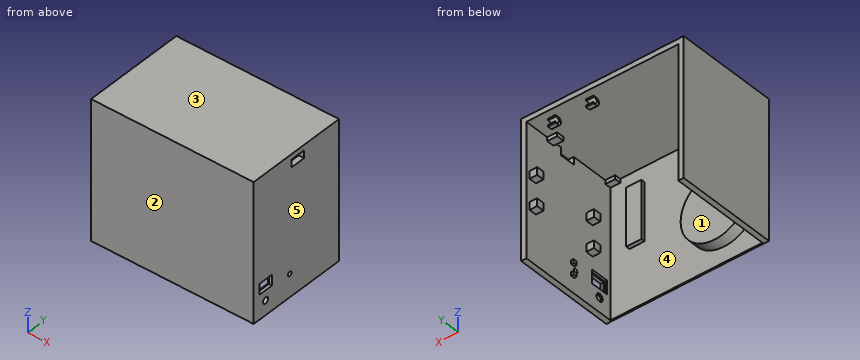
Autodesk Inventor part; units mm, degrees
ref_plane "YZ Plane" through (0, 0, 0) normal (1, 0, 0) x (0, 1, 0)
ref_plane "XY Plane" through (0, 0, 0) normal (0, 0, 1) x (1, 0, 0)
sketch "Boceto1" plane through (0, 0, 0) normal (1, 0, 0) x (0, 1, 0)
  line L0 (135, 82) -> (0, 82)
  line L1 (0, 82) -> (0, -100)
  line L2 (0, -100) -> (135, -100)
  line L3 (135, -100) -> (135, 82)
  line L4 (135, 82) -> (0, -100) construction
  line L5 (0, 82) -> (135, -100) construction
  point P0 (0, 0)
  point P1 (67.5, -9)
  dimension "d0" = 182
  dimension "d1" = 135
  dimension "d2" = 100
extrude "Extrusión1" add sketch "Boceto1" against normal blind 214
sketch "Boceto2" plane through (-214, 0, 0) normal (-1, 0, 0) x (0, 0, 1)
  line L0 (82, 135) -> (-100, 135)
  line L1 (-93, 2) -> (75, 2)
  line L2 (75, 2) -> (75, 135)
  line L3 (75, 135) -> (-93, 135)
  line L4 (-93, 135) -> (-93, 2)
  line L5 (-93, 2) -> (75, 135) construction
  line L6 (75, 2) -> (-93, 135) construction
  line L7 (-100, 0) -> (82, 0)
  line L8 (82, 0) -> (82, 135)
  line L9 (-100, 135) -> (-100, 0)
  point P0 (0, 0)
  point P1 (-9, 68.5)
  point P2 (-93, 135)
  dimension "d5" = 2
  dimension "d6" = 7
  dimension "d7" = 7
extrude "Extrusión2" cut sketch "Boceto2" against normal blind 207 contours L2 L1 L4 L0
sketch "Boceto3" plane through (0, 0, 82) normal (0, 0, 1) x (1, 0, 0)
  line L0 (-20, 0) -> (0, 0)
  line L1 (0, 0) -> (0, 10)
  line L2 (0, 10) -> (-20, 10)
  line L3 (-20, 10) -> (-20, 0)
  line L4 (-20, 0) -> (0, 10) construction
  line L5 (0, 0) -> (-20, 10) construction
  line L6 (-214, 0) -> (-194, 0)
  line L7 (-194, 0) -> (-194, 10)
  line L8 (-194, 10) -> (-214, 10)
  line L9 (-214, 10) -> (-214, 0)
  line L10 (-214, 0) -> (-194, 10) construction
  line L11 (-194, 0) -> (-214, 10) construction
  line L12 (-20, 92) -> (0, 92)
  line L13 (0, 92) -> (0, 102)
  line L14 (0, 102) -> (-20, 102)
  line L15 (-20, 102) -> (-20, 92)
  line L16 (-20, 92) -> (0, 102) construction
  line L17 (0, 92) -> (-20, 102) construction
  line L18 (-214, 0) -> (-214, 135)
  line L19 (0, 135) -> (0, 0)
  line L20 (0, 0) -> (-214, 0)
  line L21 (-214, 92) -> (-194, 92)
  line L22 (-194, 92) -> (-194, 102)
  line L23 (-194, 102) -> (-214, 102)
  line L24 (-214, 102) -> (-214, 92)
  line L25 (-214, 92) -> (-194, 102) construction
  line L26 (-194, 92) -> (-214, 102) construction
  line L27 (-214, 2) -> (-7, 2)
  point P0 (-10, 5)
  point P1 (-204, 5)
  point P2 (-10, 97)
  point P3 (-204, 97)
  point P4 (-10, 0)
  dimension "d10" = 20
  dimension "d11" = 10
  dimension "d13" = 10
  dimension "d14" = 20
  dimension "d65" = 100
extrude "Extrusión3" add sketch "Boceto3" against normal blind 12 contours L3 L2 L1 L0 | L18 L23 L22 L21 | L12 L15 L14 L13 | L6 L9 L27 L7 | L27 L9 L8 L7
sketch "Sketch4" plane through (0, 0, 0) normal (1, 0, 0) x (0, 0, -1)
  line L0 (-82, 0) -> (-82, 135)
  line L1 (-100, 90) -> (-100, 60)
  line L2 (-82, 0) -> (100, 0)
  line L3 (-75, 60) -> (-65, 60)
  line L4 (-65, 60) -> (-65, 80)
  line L5 (-65, 80) -> (-75, 80)
  line L6 (-75, 80) -> (-75, 60)
  line L7 (-75, 60) -> (-65, 80) construction
  line L8 (-65, 60) -> (-75, 80) construction
  point P0 (0, 0)
  point P1 (-70, 70)
  point P2 (-70, 60)
  dimension "d43" = 17
  dimension "d44" = 7
  dimension "d45" = 20
  dimension "d46" = 60
extrude "Extrusion4" cut sketch "Sketch4" against normal up to next
sketch "Sketch5" plane through (-7, 0, 0) normal (-1, 0, 0) x (0, 0, 1)
  line L0 (-35, 130) -> (-25, 130)
  line L1 (-25, 130) -> (-25, 120)
  line L2 (-25, 120) -> (-35, 120)
  line L3 (-35, 120) -> (-35, 130)
  line L4 (5, 130) -> (15, 130)
  line L5 (15, 130) -> (15, 120)
  line L6 (15, 120) -> (5, 120)
  line L7 (5, 120) -> (5, 130)
  line L8 (-35, 40) -> (-25, 40)
  line L9 (-25, 40) -> (-25, 30)
  line L10 (-25, 30) -> (-35, 30)
  line L11 (-35, 30) -> (-35, 40)
  line L12 (15, 40) -> (5, 40)
  line L13 (5, 40) -> (5, 30)
  line L14 (5, 30) -> (15, 30)
  line L15 (15, 30) -> (15, 40)
  line L16 (-93, 135) -> (75, 135)
  line L17 (75, 135) -> (75, 102)
  line L18 (70, 2) -> (-93, 2)
  line L19 (75, 92) -> (75, 10)
  point P0 (0, 0)
  point P1 (-30, 130)
  point P2 (-30, 30)
  point P3 (10, 130)
  point P4 (15, 125)
  dimension "d25" = 10
  dimension "d26" = 10
  dimension "d27" = 10
  dimension "d28" = 10
  dimension "d29" = 100
  dimension "d31" = 5
  dimension "d32" = 60
  dimension "d77" = 50
extrude "Extrusion5" add sketch "Sketch5" along normal blind 10
sketch "Sketch8" plane through (-7, 135, 75) normal (0, 0, -1) x (-1, 0, 0)
  line L0 (20, -20) -> (30, -20)
  line L1 (30, -20) -> (30, -10)
  line L2 (30, -10) -> (20, -10)
  line L3 (20, -10) -> (20, -20)
  line L4 (20, -20) -> (30, -10) construction
  line L5 (30, -20) -> (20, -10) construction
  line L6 (70, -20) -> (80, -20)
  line L7 (80, -20) -> (80, -10)
  line L8 (80, -10) -> (70, -10)
  line L9 (70, -10) -> (70, -20)
  line L10 (70, -20) -> (80, -10) construction
  line L11 (80, -20) -> (70, -10) construction
  line L12 (0, 0) -> (207, 0)
  line L13 (0, 0) -> (0, -33)
  point P0 (-7, -135)
  point P1 (25, -15)
  point P2 (75, -15)
  dimension "d47" = 10
  dimension "d48" = 10
  dimension "d49" = 10
  dimension "d50" = 10
  dimension "d51" = 50
  dimension "d52" = 10
  dimension "d53" = 20
extrude "Extrusion6" add sketch "Sketch8" along normal blind 10
sketch "Sketch9" plane through (-7, 0, 0) normal (-1, 0, 0) x (0, 0, 1)
  line L0 (-68, 9) -> (-54, 9)
  line L1 (-54, 9) -> (-54, 29)
  line L2 (-54, 29) -> (-68, 29)
  line L3 (-68, 29) -> (-68, 9)
  line L4 (-68, 9) -> (-54, 29) construction
  line L5 (-54, 9) -> (-68, 29) construction
  line L6 (70, 2) -> (-93, 2)
  line L7 (-93, 2) -> (-93, 135)
  circle A0 centre (-81, 19) radius 4
  point P0 (0, 0)
  point P1 (-61, 19)
  dimension "d56" = 20
  dimension "d57" = 14
  dimension "d58" = 7
  dimension "d59" = 25
  dimension "d60" = 8
  dimension "d61" = 20
  dimension "d62" = 17
extrude "Extrusion7" cut sketch "Sketch9" against normal up to next
sketch "Sketch10" plane through (-87, 115, 75) normal (-1, 0, 0) x (0, 0, 1)
  line L0 (0, 10) -> (-10, 10)
  arc A0 (-8, 10) -> (-2, 10) centre (-5, 8.1972) ccw
  line L1 (0, 20) -> (0, -13)
  point P0 (-75, -115)
  dimension "d66" = 3.5
  dimension "d67" = 2
  dimension "d68" = 2
extrude "Extrusion8" cut sketch "Sketch10" against normal up to surface (60 mm away)
sketch "Sketch11" plane through (-87, 115, 75) normal (-1, 0, 0) x (0, 0, 1)
  line L0 (-10, 10) -> (-10, 0)
  line L1 (0, 0) -> (0, 10)
  arc A0 (-10, 4.322) -> (0, 4.0877) centre (-4.9301, 7.1893) ccw
  line L2 (-10, 4.322) -> (-10, 0)
  line L3 (0, 0) -> (-10, 0)
  line L4 (0, 0) -> (0, 4.0877)
  line L5 (-10, 4.322) -> (-10, 0)
  line L6 (0, 0) -> (0, 4.0877)
  line L7 (-10, 4.322) -> (-10, 0)
  line L8 (0, 0) -> (0, 4.0877)
  line L9 (-10, 4.322) -> (-10, 0)
  line L10 (0, 0) -> (0, 4.0877)
  point P0 (-75, -115)
  point P1 (-5, 0)
  point P2 (-5.0665, 1.3663)
  dimension "d71" = 5.8246
  dimension "d73" = 4.322
  dimension "d74" = 1.3663
extrude "Extrusion9" cut sketch "Sketch11" against normal up to surface (60 mm away)
sketch "Sketch12" plane through (-214, 2, -93) normal (0, 1, 0) x (1, 0, 0)
  line L0 (162, -72) -> (182, -72)
  line L1 (182, -72) -> (182, -148)
  line L2 (182, -148) -> (162, -148)
  line L3 (162, -148) -> (162, -72)
  line L4 (162, -72) -> (182, -148) construction
  line L5 (182, -72) -> (162, -148) construction
  line L6 (207, 0) -> (207, -168)
  line L7 (207, -168) -> (0, -168)
  point P0 (214, -93)
  point P1 (172, -110)
  dimension "d78" = 76
  dimension "d79" = 20
  dimension "d80" = 25
  dimension "d81" = 20
extrude "Extrusion10" add sketch "Sketch12" along normal blind 5
sketch "Sketch13" plane through (-214, 2, -93) normal (0, 0, 1) x (1, 0, 0)
  line L0 (214, 133) -> (0, 133)
  line L1 (0, 0) -> (207, 0)
  line L2 (0, 133) -> (207, 133)
  line L3 (207, 133) -> (207, 0)
  line L4 (207, 0) -> (0, 0)
  line L5 (0, 0) -> (0, 133)
  point P0 (214, -2)
extrude "Extrusion11" cut sketch "Sketch13" against normal up to next
sketch "Sketch15" plane through (-214, 2, -100) normal (0, 1, 0) x (1, 0, 0)
  line L0 (20, -175) -> (0, -175)
  line L1 (0, 0) -> (0, -182)
  line L2 (7, -175) -> (0, -175)
  line L3 (0, -175) -> (0, 0)
  line L4 (0, 0) -> (7, 0)
  line L5 (7, 0) -> (7, -175)
  point P0 (214, -100)
  dimension "d90" = 7
extrude "Extrusion13" add sketch "Sketch15" along normal up to surface (133 mm away)
sketch "Sketch16" plane through (-194, 2, 75) normal (0, 1, 0) x (1, 0, 0)
  circle A0 centre (37.2, 110) radius 44.9
  line L0 (-13, 175) -> (-13, 0)
  line L1 (-13, 175) -> (187, 175)
  point P0 (194, 75)
  dimension "d93" = 89.8
  dimension "d94" = 50.2
  dimension "d95" = 65
extrude "Extrusion14" add sketch "Sketch16" along normal blind 15
sketch "Sketch17" plane through (-7, 0, 0) normal (-1, 0, 0) x (0, 0, 1)
  line L0 (-70, 31) -> (-52, 31)
  line L1 (-52, 31) -> (-52, 7)
  line L2 (-52, 7) -> (-70, 7)
  line L3 (-70, 7) -> (-70, 31)
  line L4 (-68, 29) -> (-54, 29)
  line L5 (-54, 29) -> (-54, 9)
  line L6 (-54, 9) -> (-68, 9)
  line L7 (-68, 9) -> (-68, 29)
  point P0 (0, 0)
  dimension "d98" = 2
  dimension "d99" = 2
  dimension "d100" = 2
  dimension "d101" = 2
extrude "Extrusion15" cut sketch "Sketch17" against normal blind 3 contours L0 L1 L2 L3 | L4 L5 L6 L7
sketch "Sketch18" plane through (-7, 0, 0) normal (-1, 0, 0) x (0, 0, 1)
  circle A0 centre (-70, 57) radius 2.95
  line L0 (70, 2) -> (-100, 2)
  line L1 (-100, 2) -> (-100, 135)
  point P0 (0, 0)
  dimension "d104" = 5.9
  dimension "d105" = 55
  dimension "d106" = 30
extrude "Extrusion16" cut sketch "Sketch18" against normal up to surface (7 mm away)
sketch "Sketch19" plane through (-7, 0, 0) normal (-1, 0, 0) x (0, 0, 1)
  line L0 (-80, 59) -> (-75, 59)
  line L1 (-75, 59) -> (-75, 64)
  line L2 (-75, 64) -> (-80, 64)
  line L3 (-80, 64) -> (-80, 59)
  line L4 (-65, 59) -> (-60, 59)
  line L5 (-60, 59) -> (-60, 64)
  line L6 (-60, 64) -> (-65, 64)
  line L7 (-65, 64) -> (-65, 59)
  circle A0 centre (-70, 57) radius 2.95
  point P0 (0, 0)
  dimension "d109" = 5
  dimension "d110" = 5
  dimension "d111" = 5
  dimension "d112" = 5
  dimension "d113" = 20
  dimension "d114" = 5
  dimension "d115" = 2
extrude "Extrusion17" add sketch "Sketch19" along normal blind 3 contours L3 L2 L1 L0 | L7 L6 L5 L4
sketch "Sketch20" plane through (-7, 0, 0) normal (-1, 0, 0) x (0, 0, 1)
  circle A0 centre (-81, 19) radius 5
  circle A1 centre (-81, 19) radius 4
  point P0 (0, 0)
  dimension "d118" = 1
extrude "Extrusion18" cut sketch "Sketch20" against normal blind 2 contours A0 | A1
ref_plane "Work Plane1" through (-207, 135, 31.25) normal (-1, 0, 0) x (0, 0, 1)
split_face "Split1"
properties part number "estructura_pieza1"
Input: part model. Units: mm. Frame: model coordinates. Face numbers are marked on the shaded views. A direction names the side the tool comes from. Round coordinates to 2 decimals unless told otherwise and drop trailing zeros. Loops run counter-clockwise (first coordinate to the right, second up) from the corner with the lowest first, then second, coordinate; pieces in that order, holes last.
1) Section query C-C on y = 43.5. Return the cut outline in (x, z), plus the area to 3 significant figures.
Ans:
outline: (-214, -100) - (-207, -100) - (-207, 75) - (-7, 75) - (-7, -100) - (0, -100) - (0, 82) - (-214, 82) - close
area: 3,950 mm2
2) Material intervals for line 1 (Y direction, x = -30, z = 70); line 2 (X direction, y = 125, z = -63.5); line 3 (Y direction, x = -2, z = -70), sorted ascending.
Ans:
line 1: y = 0 to 2, 116.37 to 119.7
line 2: x = -214 to -207, -7 to 0
line 3: y = 0 to 54.05, 59.95 to 135
3) Set-up query: the marked faces 1 and 2. Return all of +Z, -Z, +X, -X, +Y, -Y with unobstructed straight access to the full face (end or side cutting, diameter ignored); none if empty.
Ans:
face 1: -Z, +Y
face 2: +Z, -Z, +X, -X, -Y
4) Section query B-B on z = 48.5. Return the cut outline in (x, y), plus the area to 3 significant figures.
Ans:
outline: (-214, 0) - (0, 0) - (0, 135) - (-7, 135) - (-7, 2) - (-32, 2) - (-32, 7) - (-52, 7) - (-52, 2) - (-207, 2) - (-207, 135) - (-214, 135) - close
area: 2,390 mm2
5) Pin query (flat end, axial travel): pin 1 (1 mm diameter, centred on x = -82, z = 65.5, fed in from +Y); pin 2 (3 mm diameter, centred on x = -15, y = 96.5, fed in from -Z); pin 3 (1.5 mm diameter, centred on x = -50, y = 101.5, fed in from -Z); pin 4 (6 mm diameter, centred on x = -146.5, z = 50, fed in from -Y). Return the tip coordinate at first contact, or that it passes through.
Ans:
pin 1: stops at y = 125
pin 2: stops at z = 70
pin 3: stops at z = 75
pin 4: stops at y = 0
6) Section query A-A on y = 75.5. Return the cut outline in (x, z).
Ans:
outline: (-214, -100) - (-207, -100) - (-207, 75) - (0, 75) - (0, 82) - (-214, 82) - close; (-7, -100) - (0, -100) - (0, 65) - (-7, 65) - close
7) Pull-direction query (Z, two-part tool) for the marked faces 3, 4 and 5; classes: released by +Z, released by -Z, zero draft, split by the parting line, or undercut.
Ans:
face 3: released by +Z
face 4: undercut
face 5: zero draft
8) Section query D-D on x = -156.8. Return the cut outline in (y, z), plus the area to 3 significant figures.
Ans:
outline: (0, -100) - (2, -100) - (2, -79.9) - (17, -79.9) - (17, 9.9) - (2, 9.9) - (2, 75) - (135, 75) - (135, 82) - (0, 82) - close
area: 2,640 mm2
